Work out the finished part from the listing and answer in its coordinate system (mm). Face numbers are marked on the shaded views. Give positions to 0.01 mm unless a question says otherwise; leave off trailing zeros. Write each loop counter-clockwise with the first axis right and the second up, starting at its lowest first coordinate (ties: lowest second). Pieces come first, ordered by that corner, then holes. Notation, with made-up numbers: (61, 76) - (81, 76) arc R28 cw to (81, 94) - close; hole circle Ø2 at (57.25, 82.25). An arc over 180 degrees is marked (long way). Write item = value, one per line.
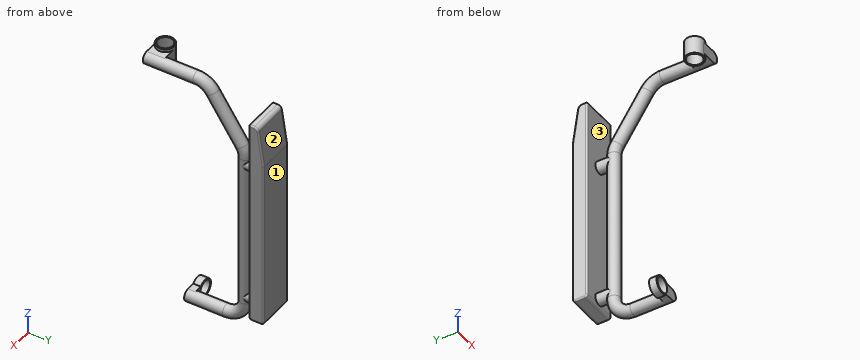
from build123d import *

# Parameters (mm, degrees)
SKETCH2_R                = 10.16
BOSS_EXTRUDE1_DEPTH      = 15.24
BOSS_EXTRUDE1_DEPTH_BACK = 15.24
SKETCH4_R                = 15.24
SKETCH5_R                = 10.16
BOSS_EXTRUDE2_DEPTH      = 15.24
SKETCH6_W                = 20.32
SKETCH6_H                = 30.48
BOSS_EXTRUDE3_DEPTH      = 25.4
SKETCH7_R                = 12.7
CUT_EXTRUDE1_DEPTH       = 461.805285208
SKETCH8_R                = 15.24
BOSS_EXTRUDE4_DEPTH      = 12.7
SKETCH10_W               = 20.32
SKETCH10_H               = 12.7
BOSS_EXTRUDE5_DEPTH      = 25.4
SKETCH11_R               = 12.7
CUT_EXTRUDE2_DEPTH       = 25.4
SKETCH12_R               = 10.16
BOSS_EXTRUDE6_DEPTH      = 25.4
BOSS_EXTRUDE7_DEPTH      = 31.75
BOSS_EXTRUDE7_DEPTH_BACK = 31.75
FILLET1_R                = 2.54
FILLET2_R                = 2.54


with BuildPart() as part:
    # Sweep1: sweep along a path in Sketch1
    with BuildLine(Plane(origin=(0, 0, 0), x_dir=(0, 0, -1), z_dir=(1, 0, 0))) as sweep1_path:
        Line((0, 0), (0, 69.32621332))
        ThreePointArc((0, 69.32621332), (3.933588394, 84.956346393), (14.797156867, 96.862523678))
        Line((14.797156867, 96.862523678), (90.432807933, 146.916310358))
        ThreePointArc((90.432807933, 146.916310358), (99.140625265, 150.999371974), (108.655651066, 152.4))
        Line((108.655651066, 152.4), (370.83999995, 152.4))
        ThreePointArc((370.83999995, 152.4), (394.188665865, 142.728665915), (403.85999995, 119.38))
        Line((403.85999995, 119.38), (403.85999995, 54.61))
    # Sketch2 → Sweep1 (sweep)
    with BuildSketch(Plane(origin=(0, 0, 0), x_dir=(1, 0, 0), z_dir=(0, 1, 0))):
        Circle(SKETCH2_R)
    sweep(path=sweep1_path.line)

    # Sketch5 → Boss-Extrude2 (add)
    with BuildSketch(Plane.XZ):
        with Locations(Location((0, 0, 0), (0, 0, 270))):
            Circle(SKETCH5_R)
    extrude(amount=BOSS_EXTRUDE2_DEPTH)



with BuildPart() as body_2:
    # Sketch4 → Boss-Extrude1 (new, two sides: drawn at the far end of the back side and taken through both)
    with BuildSketch(Plane.XY.offset(-BOSS_EXTRUDE1_DEPTH_BACK)):
        with Locations((-25.4, 0)):
            Circle(SKETCH4_R)
    extrude(amount=BOSS_EXTRUDE1_DEPTH + BOSS_EXTRUDE1_DEPTH_BACK)


with BuildPart() as part_1:
    add(part.part)

    add(body_2.part)  # Boss-Extrude3 merges body 2
    # Sketch6 → Boss-Extrude3 (add)
    with BuildSketch(Plane(origin=(0, 0, 0), x_dir=(0, 0, -1), z_dir=(1, 0, 0))):
        Rectangle(SKETCH6_W, SKETCH6_H)
    extrude(amount=-BOSS_EXTRUDE3_DEPTH)

    # Sketch7 → Cut-Extrude1 (cut, through all)
    with BuildSketch(Plane.XY.offset(15.24)):
        with Locations((-25.4, 0)):
            Circle(SKETCH7_R)
    extrude(amount=-CUT_EXTRUDE1_DEPTH, mode=Mode.SUBTRACT)



with BuildPart() as body_2_2:
    # Sketch8 → Boss-Extrude4 (new body)
    with BuildSketch(Plane(origin=(0, 54.61, 0), x_dir=(1, 0, 0), z_dir=(0, 1, 0))):
        with Locations(Location((-25.4, 403.85999995, 0), (0, 0, 270))):
            Circle(SKETCH8_R)
    extrude(amount=BOSS_EXTRUDE4_DEPTH)


with BuildPart() as part_2:
    add(part_1.part)

    add(body_2_2.part)  # Boss-Extrude5 merges body 2 2
    # Sketch10 → Boss-Extrude5 (add)
    with BuildSketch(Plane(origin=(0, 0, 0), x_dir=(0, 0, -1), z_dir=(1, 0, 0))):
        with Locations((403.85999995, 60.96)):
            Rectangle(SKETCH10_W, SKETCH10_H)
    extrude(amount=-BOSS_EXTRUDE5_DEPTH)

    # Sketch11 → Cut-Extrude2 (cut)
    with BuildSketch(Plane(origin=(0, 67.31, 0), x_dir=(1, 0, 0), z_dir=(0, 1, 0))):
        with Locations(Location((-25.4, 403.85999995, 0), (0, 0, 270))):
            Circle(SKETCH11_R)
    extrude(amount=-CUT_EXTRUDE2_DEPTH, mode=Mode.SUBTRACT)

    # Sketch12 → Boss-Extrude6 (add)
    with BuildSketch(Plane(origin=(0, 152.4, 0), x_dir=(1, 0, 0), z_dir=(0, 1, 0))):
        with Locations(Location((0, 360.410118202, 0), (0, 0, 270))):
            Circle(SKETCH12_R)
        with Locations(Location((0, 119.55398348, 0), (0, 0, 270))):
            Circle(SKETCH12_R)
    extrude(amount=BOSS_EXTRUDE6_DEPTH)

    # Sketch13 → Boss-Extrude7 (add, two sides: drawn at the far end of the back side and taken through both)
    with BuildSketch(Plane(origin=(0, 0, 0), x_dir=(0, 0, -1), z_dir=(1, 0, 0)).offset(-BOSS_EXTRUDE7_DEPTH_BACK)):
        with BuildLine():
            Line((369.685709653, 177.8), (21.679996961, 177.8))
            ThreePointArc((21.679996961, 177.8), (19.883945737, 178.543948776), (19.139996961, 180.34))
            Line((19.139996961, 180.34), (19.139996961, 186.682610789))
            ThreePointArc((19.139996961, 186.682610789), (20.983953383, 191.652693342), (25.623388191, 194.217364966))
            Line((25.623388191, 194.217364966), (85.170656017, 203.2))
            Line((85.170656017, 203.2), (369.685709653, 203.2))
            ThreePointArc((369.685709653, 203.2), (373.277812101, 201.712102448), (374.765709653, 198.12))
            Line((374.765709653, 198.12), (374.765709653, 182.88))
            ThreePointArc((374.765709653, 182.88), (373.277812101, 179.287897552), (369.685709653, 177.8))
        make_face()
    extrude(amount=BOSS_EXTRUDE7_DEPTH + BOSS_EXTRUDE7_DEPTH_BACK)

    # Fillet1
    fillet1_edges = [part_2.edges().sort_by_distance(p)[0] for p in [
        (-31.75, 177.8, -195.682853307),
        (-31.75, 198.708682483, -55.397022104),
        (-31.75, 203.2, -227.428182835),
        (-31.75, 201.712102448, -373.277812101),
        (-31.75, 190.5, -374.765709653),
        (-31.75, 179.287897552, -373.277812101),
        (-31.75, 178.543948776, -19.883945737),
        (-31.75, 183.511305395, -19.139996961),
        (-31.75, 191.652693342, -20.983953383),
        (31.75, 198.708682483, -55.397022104),
        (31.75, 191.652693342, -20.983953383),
        (31.75, 183.511305395, -19.139996961),
        (31.75, 178.543948776, -19.883945737),
        (31.75, 177.8, -195.682853307),
        (31.75, 179.287897552, -373.277812101),
        (31.75, 190.5, -374.765709653),
        (31.75, 201.712102448, -373.277812101),
        (31.75, 203.2, -227.428182835),
    ]]
    fillet(fillet1_edges, radius=FILLET1_R)

    # Fillet2
    fillet2_edges = [part_2.edges().sort_by_distance(p)[0] for p in [
        (0, 203.2, -85.170656017),
        (-31.007309319, 202.454792247, -85.226546707),
        (31.007309319, 202.454792247, -85.226546707),
    ]]
    fillet(fillet2_edges, radius=FILLET2_R)


solid = part_2.part
1. Given pin 1 (6 mm diameter, centred on x = -15, z = 5, fed in from +Y); pin 2 (9 mm diameter, centred on x = -19, z = -407, fed in from -Y); pin 3 (1 mm diameter, centred on x = -11.5, y = 65.5, fed in from -Z); pin 4 (14 mm diameter, centred on x = -3.5, y = 60.5, fed in from +Z), each flat-ended and moving along its own axis, determine where each tip first touches the part or whether it passes through.
Solution:
pin_1 = 15.24
pin_2 = through
pin_3 = -414.02
pin_4 = 10.16
2. Find section A-A, the plane z = -144.5. Give the vertices of the cut face in (x, y).
Solution:
outline = (-31.75, 180.34) arc R2.54 ccw to (-29.21, 177.8) - (29.21, 177.8) arc R2.54 ccw to (31.75, 180.34) - (31.75, 200.66) arc R2.54 ccw to (29.21, 203.2) - (-29.21, 203.2) arc R2.54 ccw to (-31.75, 200.66) - close; circle Ø20.32 at (0, 152.4)
3. Find section D-D, the plane y = 32. Give the vertices of the cut face in (x, z).
Solution:
outline = circle Ø20.32 at (0, 0)
4. For a pull along Z with two mould halves and no side action, classify the marked faces 1, 2 and 3 as pulls with the +Z half, pulls with the -Z half, needs draft (parallel to the pull), parting line crosses it, or undercut.
Solution:
face_1 = needs draft
face_2 = pulls with the +Z half
face_3 = undercut
5. Find section C-C, the plane x = 19.5. Give the vertices of the cut face in (y, z), then the cut area to 3 significant figures.
Solution:
outline = (177.8, -369.69) arc R5.08 ccw to (182.88, -374.77) - (198.12, -374.77) arc R5.08 ccw to (203.2, -369.69) - (203.2, -85.36) arc R2.54 ccw to (203.17, -84.98) - (194.22, -25.62) arc R7.62 ccw to (186.68, -19.14) - (180.34, -19.14) arc R2.54 ccw to (177.8, -21.68) - close
area = 8,680 mm^2
6. Find section B-B, the plane y = 0. Give the vertices of the cut face in (x, z), then the cut area to 3 significant figures.
Solution:
outline = (-40.64, -15.24) - (-38.1, -15.24) - (-38.1, 15.24) - (-40.64, 15.24) - close; (-12.7, -15.24) - (-10.16, -15.24) - (-10.16, -10.16) - (0, -10.16) arc R10.16 ccw to (0, 10.16) - (-10.16, 10.16) - (-10.16, 15.24) - (-12.7, 15.24) - close
area = 523 mm^2
7. Straight lines are drawn through the part: line 1 (Y direction, x = -25, z = 2); line 2 (X direction, y = 58, z = -403); line 3 (Y direction, x = -4.5, z = -167). For each, find the intervals that lie inside material, in ascending order.
Solution:
line_1 = -15.24 to -12.69, 12.69 to 15.24
line_2 = -40.62 to -38.07, -12.73 to 10.12
line_3 = 143.29 to 161.51, 177.8 to 203.2
